from build123d import *

# Parameters (mm, degrees)
F0_R     = 4.75
F1_DEPTH = 10
F2_R     = 5.5
F3_DEPTH = 5
F4_R     = 3.875
F5_DEPTH = 5.5


# Not quite as in the source:
# - a fillet or chamfer that OpenCascade refuses, or shapes differently, is made with other operations: its cross-section is extruded or revolved along the edge and cut away or added


with BuildPart() as f1:
    # F0 (on Top) → F1 (new body)
    with BuildSketch(Plane.XY):
        Circle(F0_R)
    extrude(amount=F1_DEPTH)

    # F2 (on face) → F3 (join)
    with BuildSketch(Plane.XY.offset(10)):
        Circle(F2_R)
    extrude(amount=F3_DEPTH)

    # F4 (on face) → F5 (join)
    with BuildSketch(Plane.XY.offset(15)):
        Circle(F4_R)
    extrude(amount=F5_DEPTH)

    # F6: fillet of radius 1.5 on 2 edges, made by hand

    # F6_s1 → F6_t2 (revolve, cut)
    with BuildSketch(Plane.XZ):
        with BuildLine():
            ThreePointArc((5.5, 13.5), (5.0606601718, 14.5606601718), (4, 15))
            Line((4, 15), (5.5, 15))
            Line((5.5, 15), (5.5, 13.5))
        make_face()
    revolve(axis=Axis((0, 0, 15), (0, 0, 1)), mode=Mode.SUBTRACT)

    # F6_s3 → F6_t4 (revolve, cut)
    with BuildSketch(Plane.XZ):
        with BuildLine():
            ThreePointArc((5.5, 11.2990381057), (5.2990381057, 10.5490381057), (4.75, 10))
            Line((4.75, 10), (5.5, 10))
            Line((5.5, 10), (5.5, 11.2990381057))
        make_face()
    revolve(axis=Axis((0, 0, 10), (0, 0, 1)), mode=Mode.SUBTRACT)


solid = f1.part
Design review of the part built by this model. Coordinates are the model's own, in mm. A direction names the side the tool comes from. Give positions to 0.01 mm unless a question says otherwise; leave off trailing zeros. Write each loop counter-clockwise with the first axis right and the second up, starting at its lowest first coordinate (ties: lowest second). Pieces come first, ordered by that corner, then holes. Notation, with made-up numbers: M 33.5,-31.5 L 46.5,-31.5 A17 cw 46.5,-11.5 Z; hole C -4.5,32 d10. An arc over 180 degrees is marked long. Return JSON: item names as keys, results as strings. Group by question number.
Item 1: Take a section at D-D (z = 18.75). Give the boundary of the cut face in (x, y) (3 decimals), plus the area to 3 significant figures.
Item 2: Tool access review of faces 1 (the cylindrical face through (2.192, -4.214, 4.93)), 2 (the flat face through (0, 0, 20.5)), 3 (the cylindrical face through (-0.504, 3.842, 17.712)): name each direction out of +Z, -Z, +X, -X, +Y, -Y from which nothing blocks a thin tool from reaching the whole face with its end or side.
Item 3: Take a section at A-A (x = 0). Give the boundary of the cut face in (y, z) (3 decimals).
Item 4: Wall thickness on line 1 along Y through (x, z) = (0, 7.5); line 2 along X through (y, z) = (2.75, 4); line 3 along Y through (x, z) = (-0.25, 13): over which ranges is each line inside the solid? List them lowest first.
Item 5: Clearance check with flat-ended pins moving along their axes: pin 1 Ø4 at (x, z) = (-2, 7) entering from -Y; pin 2 Ø5 at (x, z) = (-3, 3) entering from +Y; pin 3 Ø1.5 at (y, z) = (-3, 2) entering from +X. State where each tip first meets the part, or that it passes through.
Item 6: Take a section at C-C (z = 4.25). Give the boundary of the cut face in (x, y).
Return value:
{
 "1": {"outline": "C 0,0 d7.75", "area": "47.2 mm2"},
 "2": {"face 1": "-Z", "face 2": "+Z, +X, -X, +Y, -Y", "face 3": "+Z"},
 "3": {"outline": "M -5.5,11.299 A1.5 ccw -4.75,10 L -4.75,0 L 4.75,0 L 4.75,10 A1.5 ccw 5.5,11.299 L 5.5,13.5 A1.5 ccw 4,15 L 3.875,15 L 3.875,20.5 L -3.875,20.5 L -3.875,15 L -4,15 A1.5 ccw -5.5,13.5 Z"},
 "4": {"line 1": "y = -4.75 to 4.75", "line 2": "x = -3.87 to 3.87", "line 3": "y = -5.49 to 5.49"},
 "5": {"pin 1": "stops at y = -4.75", "pin 2": "stops at y = 4.72", "pin 3": "stops at x = 4.18"},
 "6": {"outline": "C 0,0 d9.5"}
}
